Input: part model. Units: mm. Frame: model coordinates. A direction names the side the tool comes from. Coordinates: 2 decimals unless noted, no trailing zeros. Loops run counter-clockwise (first coordinate to the right, second up) from the corner with the lowest first, then second, coordinate; pieces in that order, holes last.
Item 1: Ray query, line 1 along Y through (x, z) = (1.25, -4); line 2 along Y through (x, z) = (10, -1); line 3 along X through (y, z) = (-0.25, -7.5). Return the intervals inside material, ascending.
Item 2: Section A-A on z = -6.5. Return loops of the section in (x, y).
Item 3: Reachability of faces 1 (the flat face through (1.285, -1, -5)), 2 (the flat face through (5.55, -1, -5)), 3 (the flat face through (3, -1, -9.798)) from +Z, -Z, +X, -X, +Y, -Y: full face, straight path, thin tool, end or side. Return the list, or none.
Item 4: Section B-B on x = 4.5. Return loops of the section in (y, z).
Item 5: Contact query for flat-ended pins moving along their axis: P1, Ø1, axis at y = -1, z = -5.5, coming from the +X side; P2, Ø0.6, axis at y = -1, z = -7.5, coming from the -X side; P3, Ø0.6, axis at x = 4, y = -1, coming from the -Z side; P4, Ø1, axis at y = 4.5, z = -7.5, coming from the +X side. Output: stop coordinate, or through.
Item 6: Section D-D on z = -5. Return loops of the section in (x, y).
Item 7: Section C-C on y = -0.25. Return loops of the section in (x, z).
Autodesk Fusion 360 part; units mm, degrees
sketch "Sketch1" plane through (0, 0, 0) normal (0, 1, 0) x (1, 0, 0)
  line L0 (0, 0) -> (10.5, 0)
  line L1 (10.5, 0) -> (10.5, 10.5)
  line L2 (10.5, 10.5) -> (0, 10.5)
  line L3 (0, 10.5) -> (0, 0)
  dimension "d1" = 10.5
  dimension "d2" = 10.5
extrude "Extrude1" add sketch "Sketch1" along normal blind 1
sketch "Sketch2" plane through (0, 1, 0) normal (0, 1, 0) x (-1, 0, 0)
  line L0 (0, -10.5) -> (0, 0)
  line L1 (0, 0) -> (-10.5, 0)
  line L2 (-10.5, 0) -> (-10.5, -10.5)
  line L3 (-10.5, -10.5) -> (0, -10.5)
  circle A0 centre (-3.3528, -3.1902) radius 2.75
  dimension "d5" = 5.5
extrude "Extrude2" add sketch "Sketch2" along normal blind 4.3 contours A0
sketch "Sketch3" plane through (0, 0, 0) normal (0, -1, 0) x (1, 0, 0)
  line L0 (0, 0) -> (0, -10.5)
  line L1 (0, -10.5) -> (10.5, -10.5)
  line L2 (10.5, -10.5) -> (10.5, 0)
  line L3 (10.5, 0) -> (0, 0)
  line L4 (1.2846, -0.8796) -> (5.5502, -0.8796)
  line L5 (5.5502, -0.8796) -> (5.5502, -9.7985)
  line L6 (5.5502, -9.7985) -> (1.2846, -9.7985)
  line L7 (1.2846, -9.7985) -> (1.2846, -0.8796)
extrude "Extrude3" add sketch "Sketch3" along normal blind 1.2 contours L4 L5 L6 L7
Results found:
1. line 1: y = 0 to 5.3
1. line 2: y = 0 to 1
1. line 3: x = 1.28 to 5.55
2. outline: (0, 0) - (1.28, 0) - (1.28, -1.2) - (5.55, -1.2) - (5.55, 0) - (10.5, 0) - (10.5, 1) - (0, 1) - close
3. face 1: +Z, -Z, -X, -Y
3. face 2: +Z, -Z, +X, -Y
3. face 3: -Z, +X, -X, -Y
4. outline: (-1.2, -9.8) - (0, -9.8) - (0, -10.5) - (1, -10.5) - (1, -5.69) - (5.3, -5.69) - (5.3, -0.69) - (1, -0.69) - (1, 0) - (0, 0) - (0, -0.88) - (-1.2, -0.88) - close
5. P1: stops at x = 5.55
5. P2: stops at x = 1.28
5. P3: stops at z = -9.8
5. P4: passes through
6. outline: (0, 0) - (1.28, 0) - (1.28, -1.2) - (5.55, -1.2) - (5.55, 0) - (10.5, 0) - (10.5, 1) - (5.42, 1) - (5.42, 5.3) - (1.28, 5.3) - (1.28, 1) - (0, 1) - close
7. outline: (1.28, -9.8) - (5.55, -9.8) - (5.55, -0.88) - (1.28, -0.88) - close
